```python
from build123d import *

# Parameters (mm, degrees)
F0_W        = 121.92
F0_H        = 25.4
F1_DEPTH    = 66.0019
F2_W        = 203.2
F2_H        = 223.52
F3_DEPTH    = 25.4
F2_W_2      = 121.92
F2_H_2      = 132.0038
F4_DEPTH    = 127
F5_W        = 127
F5_H        = 177.8
F6_DEPTH    = 38.1
F7_R        = 38.09999
F8_T1_DEPTH = 299.2776586204
F9_W        = 177.8
F9_H        = 177.8
F10_DEPTH   = 50.8
F11_SIZE2   = 31.350927
F11_SIZE    = 177.79999
F12_W       = 177.8
F12_H       = 177.8
F13_DEPTH   = 50.8
F14_SIZE2   = 31.350927
F14_SIZE    = 177.79999
F15_R       = 6.35
F16_DEPTH   = 38.1
F17_R       = 6.35
F18_DEPTH   = 38.1
F19_R       = 6.35
F20_DEPTH   = 38.1
F21_R       = 6.35
F22_DEPTH   = 38.1


# Not quite as in the source:
# - a fillet or chamfer that OpenCascade refuses, or shapes differently, is made with other operations: its cross-section is extruded or revolved along the edge and cut away or added
# - a fillet or chamfer is up to 0.001 mm smaller than in the source, because OpenCascade refuses the exact size


with BuildPart() as f1:
    # F0 (on Front) → F1 (new body, symmetric)
    with BuildSketch(Plane.XZ):
        Rectangle(F0_W, F0_H)
    extrude(amount=F1_DEPTH, both=True)

    # F2 (on face) → F3 (join)
    with BuildSketch(Plane(origin=(0, 0, -12.7), x_dir=(1, 0, 0), z_dir=(0, 0, -1))):
        Rectangle(F2_W, F2_H)
    extrude(amount=F3_DEPTH)

    # F2 (on face) → F4 (join)
    with BuildSketch(Plane(origin=(0, 0, -12.7), x_dir=(1, 0, 0), z_dir=(0, 0, -1))):
        Rectangle(F2_W, F2_H)
        Rectangle(F2_W_2, F2_H_2, mode=Mode.SUBTRACT)
        Rectangle(F2_W_2, F2_H_2)
    extrude(amount=F4_DEPTH)

    # F5 (on face) → F6 (join)
    with BuildSketch(Plane(origin=(0, 0, -139.7), x_dir=(1, 0, 0), z_dir=(0, 0, -1))):
        Rectangle(F5_W, F5_H)
    extrude(amount=F6_DEPTH)

    # F7 (radius 38.1 in the source; OpenCascade refuses exactly that, so slightly less here)
    f7_edges = [f1.edges().sort_by_distance(p)[0] for p in [
        (0, -88.9, -177.8),
        (0, 88.9, -177.8),
    ]]
    fillet(f7_edges, radius=F7_R)

    # F8: chamfer of 38.1 x 13.8672659255 on 2 edges, made by hand

    # F8_s2 → F8_t1 (cut)
    with BuildSketch(Plane.XZ.offset(-149.6388293102)):
        Polygon((63.5, -139.7), (49.6327340745, -177.8), (63.5, -177.8), align=None)
        Polygon((-49.6327340745, -177.8), (-63.5, -139.7), (-63.5, -177.8), align=None)
    extrude(amount=F8_T1_DEPTH, mode=Mode.SUBTRACT)

    # F9 (on face) → F10 (join)
    with BuildSketch(Plane.XZ.offset(111.76)):
        with Locations((1.431e-07, -60.9599946499)):
            Rectangle(F9_W, F9_H)
    extrude(amount=F10_DEPTH)

    # F11 (size 177.8 and 31.35093717 in the source; OpenCascade refuses exactly that, so slightly less here)
    f11_edges = [f1.edges().sort_by_distance(p)[0] for p in [
        (0, -162.56, 27.940005),
    ]]
    f11_side = f1.faces().sort_by_distance((0, -162.56, -60.959995))[0]
    chamfer(f11_edges, length=F11_SIZE, length2=F11_SIZE2, reference=f11_side)

    # F12 (on face) → F13 (join)
    with BuildSketch(Plane(origin=(0, 111.76, 0), x_dir=(-1, 0, 0), z_dir=(0, 1, 0))):
        with Locations((0.0031362507, -60.9484007582)):
            Rectangle(F12_W, F12_H)
    extrude(amount=F13_DEPTH)

    # F14 (size 177.8 and 31.35093717 in the source; OpenCascade refuses exactly that, so slightly less here)
    f14_edges = [f1.edges().sort_by_distance(p)[0] for p in [
        (-0.003136, 162.56, 27.951599),
    ]]
    f14_side = f1.faces().sort_by_distance((-0.003136, 162.56, -60.948401))[0]
    chamfer(f14_edges, length=F14_SIZE, length2=F14_SIZE2, reference=f14_side)

    # F15 (on face) → F16 (join)
    with BuildSketch(Plane(origin=(0, 66.0019, 0), x_dir=(-1, 0, 0), z_dir=(0, 1, 0))):
        with Locations((101.6, -12.7)):
            Circle(F15_R)
    extrude(amount=-F16_DEPTH)

    # F17 (on face) → F18 (join)
    with BuildSketch(Plane.XZ.offset(66.0019)):
        with Locations((-101.6, -12.7)):
            Circle(F17_R)
    extrude(amount=-F18_DEPTH)

    # F19 (on face) → F20 (join)
    with BuildSketch(Plane.XZ.offset(66.0019)):
        with Locations((101.6, -12.7)):
            Circle(F19_R)
    extrude(amount=-F20_DEPTH)

    # F21 (on face) → F22 (join)
    with BuildSketch(Plane(origin=(0, 66.0019, 0), x_dir=(-1, 0, 0), z_dir=(0, 1, 0))):
        with Locations((-101.6, -12.7)):
            Circle(F21_R)
    extrude(amount=-F22_DEPTH)


solid = f1.part
```
The model under review builds one solid part; all positions refer to its coordinate system, in mm. A direction names the side the tool comes from. Coordinates: 2 decimals unless noted, no trailing zeros. Order: outer loops, then holes, each group sorted by start corner. A loop starts at its lowest first (then second) coordinate and runs counter-clockwise, first axis right, second up. Notation, with made-up numbers: M -19.5,44.5 L 7.5,44.5 A29 cw 7.5,70.5 Z; hole C 1.25,55.5 d5. An arc over 180 degrees is marked long. One line per question, with ' | ' between items.
(1) Insertion check: pin 1 (2 mm diameter, centred on y = -113, z = -135.5, fed in from -X); pin 2 (4 mm diameter, centred on x = 70, z = -41.5, fed in from +Y); pin 3 (9.5 mm diameter, centred on x = 8, y = -126, fed in from +Z). Each pin has a flat end and moves straight along its axis. Give the tip position at first contact, or say it passes through.
Geometry results:
pin 1: stops at x = -88.9 | pin 2: stops at y = 143.81 | pin 3: stops at z = 27.94
(2) The part is to be moulded in two halves that separate along Y. For faces 5 (the face through (-1, -137, -149.86)), 6 (the face through (1, 111.76, -145)), 7 (the face through (95, -111.76, -75)), 8 (the face through (-1, 66.002, 0)), say which applies: +Y half, -Y half, draft (parallel to the pull), parting line (faces both ways), or undercut.
Geometry results:
face 5: draft | face 6: undercut | face 7: -Y half | face 8: undercut
(3) For probe 1 along Y at (x, z) = (-1, -149.5); probe 2 along Z at (x, y) = (74.5, 92); probe 3 along Y at (x, z) = (52.5, -12), list the stretches that pass through material, from the lowest coordinate up. Write a range as from..to.
Geometry results:
probe 1: y = -162.5..-111.76, -87.62..87.62, 111.76..162.5 | probe 2: z = -139.7..-12.7 | probe 3: y = -138.25..-111.76, -66..66, 111.76..138.25
(4) Add section D-D, the plane z = -121. Write out the cut boundary in (x, y).
Geometry results:
outline: M -101.6,-111.76 L -88.9,-111.76 L -88.9,-157.47 L 88.9,-157.47 L 88.9,-111.76 L 101.6,-111.76 L 101.6,111.76 L 88.9,111.76 L 88.9,157.47 L -88.9,157.47 L -88.9,111.76 L -101.6,111.76 Z
(5) Add section A-A, the plane z = -145. Write out the cut boundary in (x, y).
Geometry results:
outline: M -88.9,-161.7 L 88.9,-161.7 L 88.9,-111.76 L -88.9,-111.76 Z; M -88.9,111.76 L 88.9,111.76 L 88.9,161.71 L -88.9,161.71 Z; M -61.57,-88.53 L 61.57,-88.53 L 61.57,88.53 L -61.57,88.53 Z
(6) Machinability: for faces 1 (the face through (66, -2, -139.7)), 2 (the face through (0.89, 78.04, -166.34)), 3 (the face through (88.9, -131, -82)), 4 (the face through (-103, 27.902, -11)), which of the approach directions +Z, -Z, +X, -X, +Y, -Y give a long, thin tool a straight path to every point of the face, cutting with its end or side? Answer none if there is none.
Geometry results:
face 1: -Z | face 2: -Z, +X, -X | face 3: +Z, -Z, +X, -Y | face 4: +Z, -X
(7) Add section C-C, the plane y = -46. Write out the cut boundary in (x, z).
Geometry results:
outline: M -101.6,-139.7 L -63.5,-139.7 L -49.63,-177.8 L 49.63,-177.8 L 63.5,-139.7 L 101.6,-139.7 L 101.6,-19.05 A6.35 ccw long 95.25,-12.7 L 60.96,-12.7 L 60.96,12.7 L -60.96,12.7 L -60.96,-12.7 L -95.25,-12.7 A6.35 ccw long -101.6,-19.05 Z
